Check sheet for the modelled part. Datum: model origin and axes. Units: mm. A direction names the side the tool comes from. Give positions to 0.01 mm unless a question says otherwise; leave off trailing zeros. Loops run counter-clockwise (first coordinate to the right, second up) from the corner with the lowest first, then second, coordinate; pieces in that order, holes last. Notation, with made-up numbers: (10, 48.5) - (48, 48.5) arc R27 cw to (48, 86.5) - close; hole circle Ø2 at (70.25, -31). An arc over 180 degrees is marked (long way). Answer in a Markdown table with one row per item. Add a question column.
(1) Draft check along Y on faces 1 (the face through (1.801, 2.415, 19.715)), 2 (the face through (-1.99, 5.76, 17.48)), 3 (the face through (-3, 0, 6)). Enter one of: released by +Y, released by -Y, zero draft, split by the parting line, or undercut.
(2) Sectioned sample at D-D on y = 10. Enter the section's corners in (x, z), then the cut area to 3 significant figures.
(3) Set-up check for faces 4 (the face through (-4.556, -4.636, 0.493)), 5 (the face through (-1, 9, 6)), 6 (the face through (0.243, -6.495, 14.437)), 7 (the face through (-2.75, -8, 5)): record each of +Z, -Z, +X, -X, +Y, -Y from which the full face is reachable in a straight line by a thin tool's end or side.
(4) Sectioned sample at A-A on z = 5. Enter the section's corners in (x, y), then the cut area to 3 significant figures.
(5) Thickness scan on L1, parallel to Y at x = 0, z = 1.3; L2, parallel to Z at x = 2.5, y = 8.25; L3, parallel to Z at x = 10, y = 3.25. Record the ranges inside material, lowest first.
(6) Sectioned sample at B-B on x = 7. Enter the section's corners in (y, z), then the cut area to 3 significant figures.
(7) Go/stop test with flat-tipped pins: P1, Ø1.5, axis at x = -6, z = 13, coming from the -Y side; P2, Ø1.5, axis at x = -6, z = 4, coming from the -Y side; P3, Ø5, axis at y = 0.5, z = 13, coming from the +X side. Record where each tip stops, or that it passes through.
(8) Sectioned sample at C-C on y = -7.5. Enter the section's corners in (x, z).
Autodesk Inventor part; units mm, degrees
ref_plane "YZ Plane" through (0, 0, 0) normal (1, 0, 0) x (0, 1, 0)
ref_plane "XY Plane" through (0, 0, 0) normal (0, 0, 1) x (1, 0, 0)
sketch "Sketch1" plane through (0, 0, 0) normal (0, 0, 1) x (1, 0, 0)
  line L0 (0, 0) -> (0, 7.5)
  circle A0 centre (0, 7.5) radius 1.5
  circle A1 centre (-5.3033, 5.3033) radius 1.5
  circle A2 centre (-7.5, 0) radius 1.5
  circle A3 centre (-5.3033, -5.3033) radius 1.5
  circle A4 centre (0, -7.5) radius 1.5
  circle A5 centre (5.3033, -5.3033) radius 1.5
  circle A6 centre (7.5, 0) radius 1.5
  circle A7 centre (5.3033, 5.3033) radius 1.5
  circle A8 centre (0, 0) radius 12
  dimension "d0" = 7.5
  dimension "d1" = 3
  dimension "d4" = 360
  dimension "d6" = 24
extrude "Extrusion1" add sketch "Sketch1" along normal blind 10 contours A1 | A3 | A5 | A7 | A8
sketch "Sketch2" plane through (0, 0, 0) normal (0, 0, -1) x (-1, 0, 0)
  circle A0 centre (0, 0) radius 6.5
  dimension "d9" = 13
extrude "Extrusion2" cut sketch "Sketch2" against normal blind 1
sketch "Sketch3" plane through (0, 0, 10) normal (0, 0, 1) x (1, 0, 0)
  circle A0 centre (0, 0) radius 6.5
  dimension "d12" = 13
extrude "Extrusion3" add sketch "Sketch3" along normal blind 10
sketch "Sketch4" plane through (0, 0, 10) normal (0, 0, 1) x (1, 0, 0)
  line L0 (0, 0) -> (-6.5, 0)
  circle A0 centre (0, 0) radius 6.5
  line L1 (0, 0) -> (-3.5, 0)
  line L2 (-3.5, 0) -> (3.5, 0)
  line L3 (3.5, 0) -> (3.5, -3)
  line L4 (1.75, 3.0311) -> (4.3481, 1.5311)
  line L5 (-1.75, 3.0311) -> (0.8481, 4.5311)
  line L6 (-3.5, 0) -> (-3.5, 3)
  line L7 (-1.75, -3.0311) -> (-4.3481, -1.5311)
  line L8 (1.75, -3.0311) -> (-0.8481, -4.5311)
  line L9 (0, 0) -> (0, -4.0415)
  line L10 (0, 0) -> (0, 4.0415)
  line L11 (3.5, 0) -> (3.5, 2.0207)
  line L12 (0, 4.0415) -> (1.75, 3.0311)
  line L13 (-1.75, 3.0311) -> (-3.5, 2.0207)
  line L14 (-3.5, 0) -> (-3.5, -2.0207)
  line L15 (-1.75, -3.0311) -> (0, -4.0415)
  line L16 (1.75, -3.0311) -> (3.5, -2.0207)
  line L17 (3.5, 2.0207) -> (3.5, 7.0207)
  line L18 (3.5, 7.0207) -> (-3.5, 7.0207)
  line L19 (-3.5, 7.0207) -> (-3.5, 3)
  dimension "d15" = 3.5
  dimension "d16" = 7
  dimension "d17" = 3
  dimension "d20" = 360
  dimension "d22" = 5
extrude "Extrusion4" cut sketch "Sketch4" along normal blind 6 contours L9 L15 L7 L14 L0 | L10 L12 L4 L11 L2 | L2 L3 L16 L8 L9 | L0 L6 L13 L5 L10 | L5 L13 L6 L19 A0 L17 L4 L12 | L19 L18 L17 A0
sketch "Sketch5" plane through (0, 0, 20) normal (0, 0, 1) x (1, 0, 0)
  circle A0 centre (0, 0) radius 1.5
  dimension "d25" = 3
extrude "Extrusion5" cut sketch "Sketch5" against normal up to surface (19 mm away)
sketch "Sketch6" plane through (0, 0, 20) normal (0, 0, 1) x (1, 0, 0)
  circle A0 centre (0, 0) radius 1.5
  line L0 (1.5, 0) -> (1.5, 15)
  line L1 (1.5, 0) -> (-1.5, 0)
  line L2 (-1.5, 0) -> (-1.5, 15)
  line L3 (-1.5, 15) -> (1.5, 15)
  dimension "d28" = 15
  dimension "d29" = 15
extrude "Extrusion6" cut sketch "Sketch6" against normal up to surface (4 mm away) contours A0 L2 L3 L0
fillet "Fillet1" radius 1 2 edges at (1.5, 6.3246, 18) (-1.5, 6.3246, 18)
fillet "Fillet2" radius 1 6 edges at (1.9778, 5.7518, 20) (1.5, 2.4495, 20) (0, -1.5, 20) (-1.5, 2.4495, 20) (-1.9778, 5.7518, 20) (0, -6.5, 20)
ref_plane "Work Plane1" through (0, 12, 0) normal (0, 1, 0) x (-1, 0, 0)
sketch "Sketch7" plane through (0, 12, 0) normal (0, 1, 0) x (-1, 0, 0)
  line L0 (0, 0) -> (0, 3)
  line L1 (0, 3) -> (2.75, 3)
  line L2 (2.75, 3) -> (2.75, 6)
  line L3 (2.75, 6) -> (-2.75, 6)
  line L4 (-2.75, 6) -> (-2.75, 3)
  line L5 (-2.75, 3) -> (0, 3)
  dimension "d35" = 3
  dimension "d36" = 2.75
  dimension "d37" = 3
  dimension "d38" = 5.5
extrude "Extrusion7" cut sketch "Sketch7" against normal blind 8
pattern_circular "Circular Pattern1" count 4 over 360 about axis through (0, 0, 20) along (0, 0, -1) of "Extrusion7"
sketch "Sketch8" plane through (0, 0, 10) normal (0, 0, 1) x (1, 0, 0)
  circle A0 centre (0, 0) radius 3
  dimension "d44" = 6
extrude "Extrusion8" cut sketch "Sketch8" against normal through all
properties part number "screwServo"
Reply:
| question | item | result |
|---|---|---|
| 1 | face 1 | zero draft |
| 1 | face 2 | released by +Y |
| 1 | face 3 | undercut |
| 2 | outline | (-6.63, 0) - (6.63, 0) - (6.63, 10) - (-6.63, 10) - close; hole (-2.75, 3) - (2.75, 3) - (2.75, 6) - (-2.75, 6) - close |
| 2 | area | 116 mm^2 |
| 3 | face 4 | -Z |
| 3 | face 5 | +Y |
| 3 | face 6 | +Z |
| 3 | face 7 | -Y |
| 4 | outline | (-11.68, -2.75) arc R12 ccw to (-2.75, -11.68) - (-2.75, -4) - (2.75, -4) - (2.75, -11.68) arc R12 ccw to (11.68, -2.75) - (4, -2.75) - (4, 2.75) - (11.68, 2.75) arc R12 ccw to (2.75, 11.68) - (2.75, 4) - (-2.75, 4) - (-2.75, 11.68) arc R12 ccw to (-11.68, 2.75) - (-4, 2.75) - (-4, -2.75) - close; hole circle Ø6 at (0, 0) |
| 4 | area | 250 mm^2 |
| 5 | L1 | -12 to -9, -6 to -3, 3 to 6, 9 to 12 |
| 5 | L2 | 0 to 3, 6 to 10 |
| 5 | L3 | 0 to 10 |
| 6 | outline | (-9.75, 0) - (-1.41, 0) - (-1.41, 3) - (-2.75, 3) - (-2.75, 6) - (-1.41, 6) - (-1.41, 10) - (-9.75, 10) - close; (1.41, 0) - (9.75, 0) - (9.75, 10) - (1.41, 10) - (1.41, 6) - (2.75, 6) - (2.75, 3) - (1.41, 3) - close |
| 6 | area | 159 mm^2 |
| 7 | P1 | y = -3.83 |
| 7 | P2 | y = -10.79 |
| 7 | P3 | x = 6.5 |
| 8 | outline | (-9.37, 0) - (-1.5, 0) - (-1.5, 3) - (-2.75, 3) - (-2.75, 6) - (-1.5, 6) - (-1.5, 10) - (-9.37, 10) - close; (1.5, 0) - (9.37, 0) - (9.37, 10) - (1.5, 10) - (1.5, 6) - (2.75, 6) - (2.75, 3) - (1.5, 3) - close |
